Geometry: see drawing. Coordinates: mm, zero at the bounding-box minimum. Coordinates: 2 decimals unless noted, no trailing zeros. Order: outer loops, then holes, each group sorted by start corner. A loop starts at its lowest first (then second) coordinate and runs counter-clockwise, first axis right, second up. Notation, with made-up numbers: (48, 65.25) -> (79, 65.25) arc R35 cw to (79, 100.25) -> close; hole circle Ø2 at (42, 28). An arc over 180 degrees is marked (long way). One line per item, written item: value. Start each with the question number.
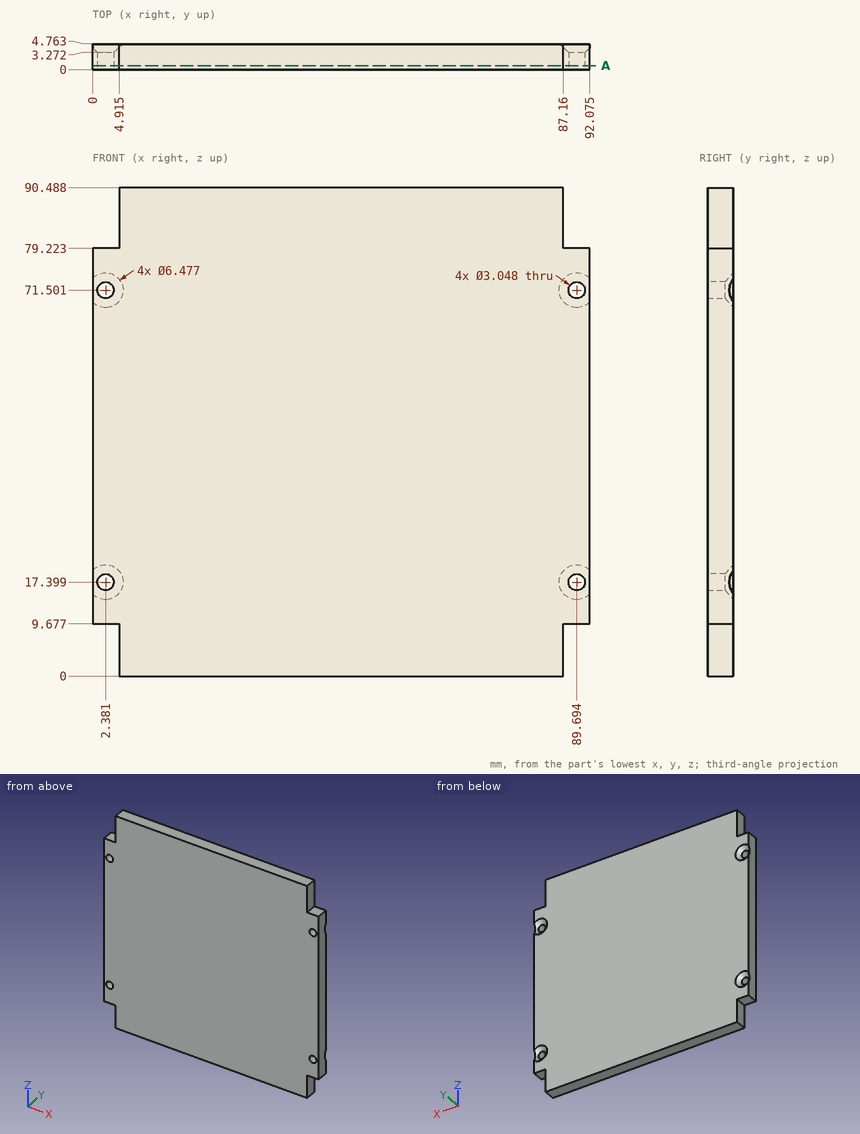
1) Ray query, line 1 along X through (y, z) = (1.75, 16) (1 decimal); line 2 along X through (y, z) = (0.8, 4) (1 decimal); line 3 along Z through (x, y) = (88, 4.35) (1 decimal). Return the intervals inside material, ascending. Write a range as from..to.
2) Section query A-A, the plane y = 0.75. Return the cut outline in (x, z) (1 decimal), plus the area to 3 significant figures.
3) Pin query (flat end, axial travel): pin 1 Ø2.5 at (x, y) = (3, 3) entering from +Z; pin 2 Ø1.4 at (y, z) = (3.5, 3.5) entering from -X (1 decimal); pin 3 Ø2.5 at (y, z) = (3, 84.5) entering from +X; pin 4 Ø1.8 at (x, z) = (2.38, 71.5) entering from -Y. Return the tip coordinate at first contact, or that it passes through.
Entries:
1. line 1: x = 0..1.8, 3..89.1, 90.3..92.1
1. line 2: x = 4.9..87.2
1. line 3: z = 9.7..15.2, 19.6..69.3, 73.7..79.2
2. outline: (0, 9.7) -> (4.9, 9.7) -> (4.9, 0) -> (87.2, 0) -> (87.2, 9.7) -> (92.1, 9.7) -> (92.1, 79.2) -> (87.2, 79.2) -> (87.2, 90.5) -> (4.9, 90.5) -> (4.9, 79.2) -> (0, 79.2) -> close; hole circle Ø3 at (2.4, 17.4); hole circle Ø3 at (2.4, 71.5); hole circle Ø3 at (89.7, 17.4); hole circle Ø3 at (89.7, 71.5)
2. area: 8,100 mm2
3. pin 1: stops at z = 79.22
3. pin 2: stops at x = 4.9
3. pin 3: stops at x = 87.16
3. pin 4: passes through
